Read the model definition and answer for the solid it produces. Units are mm, in the model's axes. A direction names the side the tool comes from. Coordinates: 2 decimals unless noted, no trailing zeros. Loops run counter-clockwise (first coordinate to the right, second up) from the corner with the lowest first, then second, coordinate; pieces in that order, holes last. Notation, with made-up numbers: (-24.75, 70.25) - (30.25, 70.25) arc R34 cw to (30.25, 106.25) - close; hole circle Ø11 at (-18.5, -22.5). An arc over 180 degrees is marked (long way). Use one line per item in the form item = value.
from build123d import *

# Parameters (mm, degrees)
SKIZZE1_W                       = 14
SKIZZE1_H                       = 14
AUFSATZ_LINEAR_AUSTRAGEN1_DEPTH = 16
FASE1_SIZE                      = 5
VERRUNDUNG2_R                   = 0.5
VERRUNDUNG3_R                   = 0.25
VERRUNDUNG4_R                   = 0.25


with BuildPart() as part:
    # Skizze1 → Aufsatz-Linear austragen1 (new body)
    with BuildSketch(Plane(origin=(0, 0, 0), x_dir=(1, 0, 0), z_dir=(0, 1, 0))):
        Rectangle(SKIZZE1_W, SKIZZE1_H)
    extrude(amount=AUFSATZ_LINEAR_AUSTRAGEN1_DEPTH)

    # Skizze6 → Schnitt-Rotation4 (revolve, cut)
    with BuildSketch(Plane(origin=(0, 0, 0), x_dir=(0, 0, -1), z_dir=(1, 0, 0))):
        Polygon((6.25, 16), (13.25, 16), (13.25, 9), (4, 9), (4, 13), (6.25, 13), align=None)
    revolve(axis=Axis((0, 0, 0), (0, 1, 0)), mode=Mode.SUBTRACT)

    # Fase1
    # the kernel refuses this chamfer: 5 mm, written as the material it takes off along each edge
    with BuildSketch(Plane(origin=(-7, 9, 19.85841494), x_dir=(0.9996219169112968, 0.027495876610586317, 0), z_dir=(0, 0, -1))) as fase1_piece_1_section:
        Polygon((FASE1_SIZE * 0.999621916911, FASE1_SIZE * 0.0274958766106), (-FASE1_SIZE * 0.0274958766106, FASE1_SIZE * 0.999621916911), (0, 0), align=None)
    fase1_piece_1 = extrude(amount=39.71682988, mode=Mode.PRIVATE)
    fase1_piece_1 = fase1_piece_1 - Plane(origin=(0, 7.328837599, 0), x_dir=(0, 0, -1), z_dir=(0, 1, 0)) * Cylinder(4, 100, mode=Mode.PRIVATE)
    add(fase1_piece_1, mode=Mode.SUBTRACT)
    with BuildSketch(Plane(origin=(-19.85841494, 9, -7), x_dir=(0, -0.9996219169112968, -0.027495876610586317), z_dir=(1, 0, 0))) as fase1_piece_2_section:
        Polygon((FASE1_SIZE * 0.999621916911, -FASE1_SIZE * 0.0274958766106), (-FASE1_SIZE * 0.0274958766106, -FASE1_SIZE * 0.999621916911), (0, 0), align=None)
    fase1_piece_2 = extrude(amount=39.71682988, mode=Mode.PRIVATE)
    fase1_piece_2 = fase1_piece_2 - Plane(origin=(0, 7.328837565, 0), x_dir=(0, 0, -1), z_dir=(0, 1, 0)) * Cylinder(4, 100, mode=Mode.PRIVATE)
    add(fase1_piece_2, mode=Mode.SUBTRACT)
    with BuildSketch(Plane(origin=(7, 9, -19.85841494), x_dir=(0.027495876610586317, -0.9996219169112968, 0), z_dir=(0, 0, 1))) as fase1_piece_3_section:
        Polygon((FASE1_SIZE * 0.999621916911, -FASE1_SIZE * 0.0274958766106), (-FASE1_SIZE * 0.0274958766106, -FASE1_SIZE * 0.999621916911), (0, 0), align=None)
    fase1_piece_3 = extrude(amount=39.71682988, mode=Mode.PRIVATE)
    fase1_piece_3 = fase1_piece_3 - Plane(origin=(0, 7.328837548, 0), x_dir=(0, 0, -1), z_dir=(0, 1, 0)) * Cylinder(4, 100, mode=Mode.PRIVATE)
    add(fase1_piece_3, mode=Mode.SUBTRACT)
    with BuildSketch(Plane(origin=(19.85841494, 9, 7), x_dir=(0, 0.027495876610586317, -0.9996219169112968), z_dir=(-1, 0, 0))) as fase1_piece_4_section:
        Polygon((FASE1_SIZE * 0.999621916911, FASE1_SIZE * 0.0274958766106), (-FASE1_SIZE * 0.0274958766106, FASE1_SIZE * 0.999621916911), (0, 0), align=None)
    fase1_piece_4 = extrude(amount=39.71682988, mode=Mode.PRIVATE)
    fase1_piece_4 = fase1_piece_4 - Plane(origin=(0, 7.328837599, 0), x_dir=(0, 0, -1), z_dir=(0, 1, 0)) * Cylinder(4, 100, mode=Mode.PRIVATE)
    add(fase1_piece_4, mode=Mode.SUBTRACT)

    # Verrundung2
    verrundung2_edges = [part.edges().sort_by_distance(p)[0] for p in [
        (0, 16, 6.25),
    ]]
    fillet(verrundung2_edges, radius=VERRUNDUNG2_R)

    # Verrundung3
    verrundung3_edges = [part.edges().sort_by_distance(p)[0] for p in [
        (-7, 4, 0),
        (0, 4, -7),
        (7, 4, 0),
        (0, 4, 7),
    ]]
    fillet(verrundung3_edges, radius=VERRUNDUNG3_R)

    # Verrundung4
    verrundung4_edges = [part.edges().sort_by_distance(p)[0] for p in [
        (0, 13, 6.25),
    ]]
    fillet(verrundung4_edges, radius=VERRUNDUNG4_R)


solid = part.part
Item 1: The part is cut by section A-A on x = 0. Give the vertices of the cut face in (y, z).
Results below:
outline = (0, -7) - (3.9, -7) arc R0.25 ccw to (4.07, -6.93) - (7, -4) - (13, -4) - (13, -6) arc R0.25 ccw to (13.25, -6.25) - (15.5, -6.25) arc R0.5 ccw to (16, -5.75) - (16, 5.75) arc R0.5 ccw to (15.5, 6.25) - (13.25, 6.25) arc R0.25 ccw to (13, 6) - (13, 4) - (7, 4) - (4.07, 6.93) arc R0.25 ccw to (3.9, 7) - (0, 7) - close
Item 2: For a pull along Y with two mould halves and no side action, classify faces 3 (the cylindrical face through (-1.346, 10.639, -3.767)), 4 (the flat face through (0, 0, 0)), 5 (the flat face through (0, 6, -5)), 6 (the cylindrical face through (-1.88, 14.39, -5.96)) as +Y half, -Y half, draft (parallel to the pull), parting line (faces both ways), or undercut.
Results below:
face_3 = undercut
face_4 = -Y half
face_5 = undercut
face_6 = draft
Item 3: Which of the six approach directions +Z, -Z, +X, -X, +Y, -Y give full straight-line access (tool end or side, diameter ignored) to faces 1 (the flat face through (-7, 2, 0)), 2 (the flat face through (3.92, 13, -1.42))?
Results below:
face_1 = +Z, -Z, -X, +Y, -Y
face_2 = none
Item 4: Find the intervals of material crossed by L1, parallel to Y at x = 3.5, z = 4; L2, parallel to Y at x = -1.5, z = -5; L3, parallel to Z at x = -2.75, y = 5, in increasing order.
Results below:
L1 = 0 to 7, 13 to 16
L2 = 0 to 6, 13 to 16
L3 = -6 to 6
Item 5: The part is cut by section B-B on z = 0. Give the vertices of the cut face in (x, y).
Results below:
outline = (-7, 0) - (7, 0) - (7, 3.9) arc R0.25 ccw to (6.93, 4.07) - (4, 7) - (4, 13) - (6, 13) arc R0.25 ccw to (6.25, 13.25) - (6.25, 15.5) arc R0.5 ccw to (5.75, 16) - (-5.75, 16) arc R0.5 ccw to (-6.25, 15.5) - (-6.25, 13.25) arc R0.25 ccw to (-6, 13) - (-4, 13) - (-4, 7) - (-6.93, 4.07) arc R0.25 ccw to (-7, 3.9) - close
Item 6: Each of these flat-tipped pins is pushed along its axis until it touches: P1, Ø1, axis at x = 0, y = 13.5, coming from the +Z side; P2, Ø2, axis at y = 5, z = 2, coming from the -X side; P3, Ø1, axis at x = 5.5, z = -5, coming from the +Y side. Where does it stop, or does it pass through?
Results below:
P1 = 6.25
P2 = -6.98
P3 = 6
Item 7: The part is cut by section C-C on y = 10.25. Give the vertices of the cut face in (x, z), plus the area to 3 significant figures.
Results below:
outline = circle Ø8 at (0, 0)
area = 50.3 mm²
